Here's how the part is built. I have some questions about the finished solid (model axes, mm). A direction names the side the tool comes from. Coordinates: 2 decimals unless noted, no trailing zeros. Loops run counter-clockwise (first coordinate to the right, second up) from the corner with the lowest first, then second, coordinate; pieces in that order, holes last. Notation, with made-up numbers: M 88,56 L 120,56 A10 cw 120,62 Z; hole C 47,18 d6. An arc over 180 degrees is marked long. Use one line per item in the form item = value. Start each with the question number.
(1) Will these pins go through, and if not, where does the flat tip stop? P1, Ø2, axis at x = 61, z = 41.5, coming from the +Y side; P2, Ø2.5, axis at x = 59.5, y = 20, coming from the -Z side; P3, Ø6, axis at y = 11, z = 12, coming from the +X side.
(2) Please list where these lines run through material, in increasing order: L1, parallel to Y at x = -51, z = 25.5; L2, parallel to Z at x = 43.5, y = 12; L3, parallel to Z at x = -8, y = 13.5.
(3) Imagine slicing it at B-B, the plane x = 33. Please give me the cut outline in (y, z), and give its area (3 significant figures).
(4) Thinking about a two-plate mould opening in X: for faces 6 (the cylindrical face through (26.535, 17.29, 35.91)), 7 (the flat face through (53, 27.5, -40)), which applies, +X half, -X half, draft (parallel to the pull), parting line (faces both ways), or undercut?
(5) Imagine slicing it at A-A, the plane z = -16.5. Please give me the cut outline in (x, y).
(6) On a 3-axis mill with a long thin cutter (end or side, diameter ignored), from which of +Z, -Z, +X, -X, +Y, -Y can I reach the whole of each face in a straight line? I mean faces 1 (the flat face through (60, 17, 41.914)), 2 (the flat face through (60, 17, -39.914)), 3 (the flat face through (53, 7.5, -40)), 4 (the cylindrical face through (-53.8, 17.29, -12.64)), 5 (the flat face through (1, 17, 42.5)). Say none if no direction works.
(7) Imagine slicing it at C-C, the plane y = 29. State how many separate pieces and enclosed holes the cut face has, and give its area (3 significant figures).
(8) Imagine slicing it at D-D, the plane x = 0. Please give me the cut outline in (y, z).
```python
from build123d import *

# Parameters (mm, degrees)
SKETCH_1_W          = 115
SKETCH_1_H          = 90
EXTRUDE_1_DEPTH     = 35
SKETCH_2_W          = 85
SKETCH_2_H          = 30
CUT_EXTRUDE_1_DEPTH = 129.35497653
SKETCH_3_W          = 4
SKETCH_3_H          = 20
EXTRUDE_2_DEPTH     = 10
SKETCH_4_W          = 2
SKETCH_4_H          = 17.171572876
EXTRUDE_3_DEPTH     = 5
SKETCH_5_R          = 2
SKETCH_5_R_2        = 10
EXTRUDE_4_DEPTH     = 32


with BuildPart() as part:
    # Эскиз1 → Бобышка-Вытянуть1 (new body)
    with BuildSketch(Plane(origin=(0, 0, 0), x_dir=(1, 0, 0), z_dir=(0, 1, 0))):
        Rectangle(SKETCH_1_W, SKETCH_1_H)
    extrude(amount=EXTRUDE_1_DEPTH)

    # Эскиз2 → Вырез-Вытянуть1 (cut, through all)
    with BuildSketch(Plane(origin=(57.5, 0, 0), x_dir=(0, 0, -1), z_dir=(1, 0, 0))):
        with Locations((0, 17.5)):
            Rectangle(SKETCH_2_W, SKETCH_2_H)
    extrude(amount=-CUT_EXTRUDE_1_DEPTH, mode=Mode.SUBTRACT)

    # Эскиз3 → Бобышка-Вытянуть2 (add)
    with BuildSketch(Plane(origin=(57.5, 0, 0), x_dir=(0, 0, -1), z_dir=(1, 0, 0))):
        with Locations((40.5, 17.5)):
            Rectangle(SKETCH_3_W, SKETCH_3_H)
        with Locations((-40.5, 17.5)):
            Rectangle(SKETCH_3_W, SKETCH_3_H)
    extrude(amount=-EXTRUDE_2_DEPTH)

    # Эскиз4 → Бобышка-Вытянуть3 (add)
    with BuildSketch(Plane(origin=(57.5, 0, 0), x_dir=(0, 0, -1), z_dir=(1, 0, 0))):
        with Locations((40.914213562, 17.5)):
            Rectangle(SKETCH_4_W, SKETCH_4_H)
        with Locations((-40.914213562, 17.5)):
            Rectangle(SKETCH_4_W, SKETCH_4_H)
    extrude(amount=EXTRUDE_3_DEPTH)

    # Эскиз5 → Бобышка-Вытянуть4 (add)
    with BuildSketch(Plane(origin=(0, 2.5, 0), x_dir=(1, 0, 0), z_dir=(0, 1, 0))):
        with Locations(Location((-52.113626613, 34.564029455, 0), (0, 0, 90))):
            Circle(SKETCH_5_R)
        with Locations(Location((-52.113626613, 11.564029455, 0), (0, 0, 90))):
            Circle(SKETCH_5_R)
        with Locations(Location((-52.113626613, -11.435970545, 0), (0, 0, 90))):
            Circle(SKETCH_5_R)
        with Locations(Location((-52.113626613, -34.435970545, 0), (0, 0, 90))):
            Circle(SKETCH_5_R)
        with Locations(Location((53.054505716, 34.564029455, 0), (0, 0, 90))):
            Circle(SKETCH_5_R)
        with Locations(Location((53.054505716, 11.564029455, 0), (0, 0, 90))):
            Circle(SKETCH_5_R)
        with Locations(Location((53.054505716, -11.435970545, 0), (0, 0, 90))):
            Circle(SKETCH_5_R)
        with Locations(Location((53.054505716, -34.435970545, 0), (0, 0, 90))):
            Circle(SKETCH_5_R)
        with Locations(Location((-12.113626613, 34.564029455, 0), (0, 0, 90))):
            Circle(SKETCH_5_R)
        with Locations(Location((27.886373387, 34.564029455, 0), (0, 0, 90))):
            Circle(SKETCH_5_R)
        with Locations(Location((-12.113626613, -34.435970545, 0), (0, 0, 90))):
            Circle(SKETCH_5_R)
        with Locations(Location((27.886373387, -34.435970545, 0), (0, 0, 90))):
            Circle(SKETCH_5_R)
        with Locations(Location((0, 0, 0), (0, 0, 90))):
            Circle(SKETCH_5_R_2)
    extrude(amount=EXTRUDE_4_DEPTH)


solid = part.part
```
Answer:
q1.P1 = 26.09
q1.P2 = -41.91
q1.P3 = 55.05
q2.L1 = 0 to 2.5, 32.5 to 35
q2.L2 = -45 to -42.5, 42.5 to 45
q2.L3 = -45 to -42.5, -6 to 6, 42.5 to 45
q3.outline = M 0,-45 L 35,-45 L 35,45 L 0,45 Z; hole M 2.5,-42.5 L 32.5,-42.5 L 32.5,42.5 L 2.5,42.5 Z
q3.area = 600 mm²
q4.face_6 = undercut
q4.face_7 = draft
q5.outline = M -57.5,0 L 57.5,0 L 57.5,2.5 L -57.5,2.5 Z; M -57.5,32.5 L 57.5,32.5 L 57.5,35 L -57.5,35 Z
q6.face_1 = +Z, +X, +Y, -Y
q6.face_2 = +X, +Y, -Y
q6.face_3 = +X, -X
q6.face_4 = none
q6.face_5 = -X
q7.separate_pieces = 15
q7.enclosed_holes = 0
q7.area = 1,040 mm²
q8.outline = M 0,-45 L 35,-45 L 35,45 L 0,45 Z; hole M 2.5,-42.5 L 32.5,-42.5 L 32.5,-10 L 2.5,-10 Z; hole M 2.5,10 L 32.5,10 L 32.5,42.5 L 2.5,42.5 Z
